from build123d import *

# Parameters (mm, degrees)
SKETCH_1_R          = 2
SKETCH_1_W          = 3
SKETCH_1_H          = 50
EXTRUDE_1_DEPTH     = 10
SKETCH_2_R          = 2
CUT_EXTRUDE_1_DEPTH = 513.83835495


with BuildPart() as part:
    # 스케치1 → 보스-돌출1 (new body)
    with BuildSketch(Plane(origin=(0, 0, 0), x_dir=(1, 0, 0), z_dir=(0, 1, 0))):
        Polygon((-478.203072248, 175), (-448.173072248, 175), (-448.173072248, 185), (-398.173072248, 185), (-398.173072248, 175), (-348.173072248, 175), (-348.173072248, 185), (-298.173072248, 185), (-298.173072248, 175), (-248.173072248, 175), (-248.173072248, 185), (-198.173072248, 185), (-198.173072248, 175), (-148.173072248, 175), (-148.173072248, 185), (-98.173072248, 185), (-98.173072248, 175), (-48.173072248, 175), (-48.173072248, 185), (1.826927752, 185), (1.826927752, 175), (51.826927752, 175), (51.826927752, 185), (101.826927752, 185), (101.826927752, 175), (151.826927752, 175), (151.826927752, 185), (201.826927752, 185), (201.826927752, 175), (207.156927752, 175), (207.156927752, -175), (201.826927752, -175), (201.826927752, -185), (151.826927752, -185), (151.826927752, -175), (101.826927752, -175), (101.826927752, -185), (51.826927752, -185), (51.826927752, -175), (1.826927752, -175), (1.826927752, -185), (-48.173072248, -185), (-48.173072248, -175), (-98.173072248, -175), (-98.173072248, -185), (-148.173072248, -185), (-148.173072248, -175), (-198.173072248, -175), (-198.173072248, -185), (-248.173072248, -185), (-248.173072248, -175), (-298.173072248, -175), (-298.173072248, -185), (-348.173072248, -185), (-348.173072248, -175), (-398.173072248, -175), (-398.173072248, -185), (-448.173072248, -185), (-448.173072248, -175), (-478.203072248, -175), align=None)
        with Locations(Location((-340.173072248, 169, 0), (0, 0, 270))):
            Circle(SKETCH_1_R, mode=Mode.SUBTRACT)
        with Locations(Location((-306.173072248, 169, 0), (0, 0, 270))):
            Circle(SKETCH_1_R, mode=Mode.SUBTRACT)
        with Locations(Location((-290.173072248, 169, 0), (0, 0, 270))):
            Circle(SKETCH_1_R, mode=Mode.SUBTRACT)
        with Locations(Location((-256.173072248, 169, 0), (0, 0, 270))):
            Circle(SKETCH_1_R, mode=Mode.SUBTRACT)
        with Locations(Location((-240.173072248, 169, 0), (0, 0, 270))):
            Circle(SKETCH_1_R, mode=Mode.SUBTRACT)
        with Locations(Location((-206.173072248, 169, 0), (0, 0, 270))):
            Circle(SKETCH_1_R, mode=Mode.SUBTRACT)
        with Locations(Location((-190.173072248, 169, 0), (0, 0, 270))):
            Circle(SKETCH_1_R, mode=Mode.SUBTRACT)
        with Locations(Location((-156.173072248, 169, 0), (0, 0, 270))):
            Circle(SKETCH_1_R, mode=Mode.SUBTRACT)
        with Locations(Location((-140.173072248, 169, 0), (0, 0, 270))):
            Circle(SKETCH_1_R, mode=Mode.SUBTRACT)
        with Locations(Location((-106.173072248, 169, 0), (0, 0, 270))):
            Circle(SKETCH_1_R, mode=Mode.SUBTRACT)
        with Locations(Location((-90.173072248, 169, 0), (0, 0, 270))):
            Circle(SKETCH_1_R, mode=Mode.SUBTRACT)
        with Locations(Location((-56.173072248, 169, 0), (0, 0, 270))):
            Circle(SKETCH_1_R, mode=Mode.SUBTRACT)
        with Locations(Location((-40.173072248, 169, 0), (0, 0, 270))):
            Circle(SKETCH_1_R, mode=Mode.SUBTRACT)
        with Locations(Location((-6.173072248, 169, 0), (0, 0, 270))):
            Circle(SKETCH_1_R, mode=Mode.SUBTRACT)
        with Locations(Location((9.826927752, 169, 0), (0, 0, 270))):
            Circle(SKETCH_1_R, mode=Mode.SUBTRACT)
        with Locations(Location((43.826927752, 169, 0), (0, 0, 270))):
            Circle(SKETCH_1_R, mode=Mode.SUBTRACT)
        with Locations(Location((59.826927752, 169, 0), (0, 0, 270))):
            Circle(SKETCH_1_R, mode=Mode.SUBTRACT)
        with Locations(Location((93.826927752, 169, 0), (0, 0, 270))):
            Circle(SKETCH_1_R, mode=Mode.SUBTRACT)
        with Locations(Location((93.826927752, -169, 0), (0, 0, 90))):
            Circle(SKETCH_1_R, mode=Mode.SUBTRACT)
        with Locations(Location((59.826927752, -169, 0), (0, 0, 90))):
            Circle(SKETCH_1_R, mode=Mode.SUBTRACT)
        with Locations(Location((43.826927752, -169, 0), (0, 0, 90))):
            Circle(SKETCH_1_R, mode=Mode.SUBTRACT)
        with Locations(Location((9.826927752, -169, 0), (0, 0, 90))):
            Circle(SKETCH_1_R, mode=Mode.SUBTRACT)
        with Locations(Location((-6.173072248, -169, 0), (0, 0, 90))):
            Circle(SKETCH_1_R, mode=Mode.SUBTRACT)
        with Locations(Location((-40.173072248, -169, 0), (0, 0, 90))):
            Circle(SKETCH_1_R, mode=Mode.SUBTRACT)
        with Locations(Location((-56.173072248, -169, 0), (0, 0, 90))):
            Circle(SKETCH_1_R, mode=Mode.SUBTRACT)
        with Locations(Location((-90.173072248, -169, 0), (0, 0, 90))):
            Circle(SKETCH_1_R, mode=Mode.SUBTRACT)
        with Locations(Location((-106.173072248, -169, 0), (0, 0, 90))):
            Circle(SKETCH_1_R, mode=Mode.SUBTRACT)
        with Locations(Location((-140.173072248, -169, 0), (0, 0, 90))):
            Circle(SKETCH_1_R, mode=Mode.SUBTRACT)
        with Locations(Location((-156.173072248, -169, 0), (0, 0, 90))):
            Circle(SKETCH_1_R, mode=Mode.SUBTRACT)
        with Locations(Location((-190.173072248, -169, 0), (0, 0, 90))):
            Circle(SKETCH_1_R, mode=Mode.SUBTRACT)
        with Locations(Location((-206.173072248, -169, 0), (0, 0, 90))):
            Circle(SKETCH_1_R, mode=Mode.SUBTRACT)
        with Locations(Location((-240.173072248, -169, 0), (0, 0, 90))):
            Circle(SKETCH_1_R, mode=Mode.SUBTRACT)
        with Locations(Location((-256.173072248, -169, 0), (0, 0, 90))):
            Circle(SKETCH_1_R, mode=Mode.SUBTRACT)
        with Locations(Location((-290.173072248, -169, 0), (0, 0, 90))):
            Circle(SKETCH_1_R, mode=Mode.SUBTRACT)
        with Locations(Location((-306.173072248, -169, 0), (0, 0, 90))):
            Circle(SKETCH_1_R, mode=Mode.SUBTRACT)
        with Locations(Location((-340.173072248, -169, 0), (0, 0, 90))):
            Circle(SKETCH_1_R, mode=Mode.SUBTRACT)
        with Locations(Location((-388.173072248, -163, 0), (0, 0, 270))):
            Circle(SKETCH_1_R, mode=Mode.SUBTRACT)
        with Locations(Location((-358.173072248, -163, 0), (0, 0, 270))):
            Circle(SKETCH_1_R, mode=Mode.SUBTRACT)
        with Locations(Location((-388.173072248, -148, 0), (0, 0, 270))):
            Circle(SKETCH_1_R, mode=Mode.SUBTRACT)
        with Locations(Location((-358.173072248, -148, 0), (0, 0, 270))):
            Circle(SKETCH_1_R, mode=Mode.SUBTRACT)
        with Locations(Location((-388.173072248, -133, 0), (0, 0, 270))):
            Circle(SKETCH_1_R, mode=Mode.SUBTRACT)
        with Locations(Location((-358.173072248, -133, 0), (0, 0, 270))):
            Circle(SKETCH_1_R, mode=Mode.SUBTRACT)
        with Locations(Location((-358.173072248, 163, 0), (0, 0, 90))):
            Circle(SKETCH_1_R, mode=Mode.SUBTRACT)
        with Locations(Location((-388.173072248, 163, 0), (0, 0, 90))):
            Circle(SKETCH_1_R, mode=Mode.SUBTRACT)
        with Locations(Location((-388.173072248, 148, 0), (0, 0, 90))):
            Circle(SKETCH_1_R, mode=Mode.SUBTRACT)
        with Locations(Location((-358.173072248, 148, 0), (0, 0, 90))):
            Circle(SKETCH_1_R, mode=Mode.SUBTRACT)
        with Locations(Location((-358.173072248, 133, 0), (0, 0, 90))):
            Circle(SKETCH_1_R, mode=Mode.SUBTRACT)
        with Locations(Location((-388.173072248, 133, 0), (0, 0, 90))):
            Circle(SKETCH_1_R, mode=Mode.SUBTRACT)
        with Locations(Location((111.826927752, -163, 0), (0, 0, 270))):
            Circle(SKETCH_1_R, mode=Mode.SUBTRACT)
        with Locations(Location((141.826927752, -163, 0), (0, 0, 270))):
            Circle(SKETCH_1_R, mode=Mode.SUBTRACT)
        with Locations(Location((111.826927752, -148, 0), (0, 0, 270))):
            Circle(SKETCH_1_R, mode=Mode.SUBTRACT)
        with Locations(Location((141.826927752, -148, 0), (0, 0, 270))):
            Circle(SKETCH_1_R, mode=Mode.SUBTRACT)
        with Locations(Location((111.826927752, -133, 0), (0, 0, 270))):
            Circle(SKETCH_1_R, mode=Mode.SUBTRACT)
        with Locations(Location((141.826927752, -133, 0), (0, 0, 270))):
            Circle(SKETCH_1_R, mode=Mode.SUBTRACT)
        with Locations(Location((141.826927752, 133, 0), (0, 0, 90))):
            Circle(SKETCH_1_R, mode=Mode.SUBTRACT)
        with Locations(Location((141.826927752, 148, 0), (0, 0, 90))):
            Circle(SKETCH_1_R, mode=Mode.SUBTRACT)
        with Locations(Location((141.826927752, 163, 0), (0, 0, 90))):
            Circle(SKETCH_1_R, mode=Mode.SUBTRACT)
        with Locations(Location((111.826927752, 163, 0), (0, 0, 90))):
            Circle(SKETCH_1_R, mode=Mode.SUBTRACT)
        with Locations(Location((111.826927752, 148, 0), (0, 0, 90))):
            Circle(SKETCH_1_R, mode=Mode.SUBTRACT)
        with Locations(Location((111.826927752, 133, 0), (0, 0, 90))):
            Circle(SKETCH_1_R, mode=Mode.SUBTRACT)
        with Locations((-166.673072248, 100)):
            Rectangle(SKETCH_1_W, SKETCH_1_H, mode=Mode.SUBTRACT)
        with Locations((-166.673072248, 0)):
            Rectangle(SKETCH_1_W, SKETCH_1_H, mode=Mode.SUBTRACT)
        with Locations((-166.673072248, -100)):
            Rectangle(SKETCH_1_W, SKETCH_1_H, mode=Mode.SUBTRACT)
        with Locations((-399.473072248, 100)):
            Rectangle(SKETCH_1_W, SKETCH_1_H, mode=Mode.SUBTRACT)
        with Locations((-399.473072248, 0)):
            Rectangle(SKETCH_1_W, SKETCH_1_H, mode=Mode.SUBTRACT)
        with Locations((-399.473072248, -100)):
            Rectangle(SKETCH_1_W, SKETCH_1_H, mode=Mode.SUBTRACT)
    extrude(amount=EXTRUDE_1_DEPTH)

    # 스케치2 → 컷-돌출1 (cut, through all)
    with BuildSketch(Plane(origin=(0, 10, 0), x_dir=(1, 0, 0), z_dir=(0, 1, 0))):
        with Locations(Location((137.156927752, 30, 0), (0, 0, 270))):
            Circle(SKETCH_2_R)
        with Locations(Location((187.156927752, 30, 0), (0, 0, 270))):
            Circle(SKETCH_2_R)
        with Locations(Location((-65.173072248, 30, 0), (0, 0, 270))):
            Circle(SKETCH_2_R)
        with Locations(Location((-65.173072248, -30, 0), (0, 0, 90))):
            Circle(SKETCH_2_R)
        with Locations(Location((187.156927752, -30, 0), (0, 0, 90))):
            Circle(SKETCH_2_R)
        with Locations(Location((137.156927752, -30, 0), (0, 0, 90))):
            Circle(SKETCH_2_R)
    extrude(amount=-CUT_EXTRUDE_1_DEPTH, mode=Mode.SUBTRACT)


solid = part.part
Can you work these out from the model? Positions are in its coordinate system, mm. Give positions to 0.01 mm unless a question says otherwise; leave off trailing zeros. Write each loop counter-clockwise with the first axis right and the second up, starting at its lowest first coordinate (ties: lowest second). Pieces come first, ordered by that corner, then holes. Notation, with made-up numbers: (43.25, 0.25) -> (85.25, 0.25) arc R19 cw to (85.25, 21.25) -> close; hole circle Ø1 at (16.25, 39). An arc over 180 degrees is marked (long way). Answer as a JSON object with one key per item and string values. Group by question number.
Item 1: I'm going to push flat-ended pins straight in: P1, Ø1.5, axis at x = 126.5, y = 7, coming from the +Z side; P2, Ø5, axis at y = 5.5, z = -178.5, coming from the +X side. Where does each tip first touch, or does it pass through?
Item 2: Please list where these lines run through material, in increasing order: line 1 (X direction, y = 6.25, z = 99); line 2 (X direction, y = 5.5, z = -133); line 3 (Z direction, x = 150.5, y = 5.5). Write a range as [from, to].
Item 3: Suppose I cut it at A-A (x = -377). Please give me the cut outline in (y, z).
Item 4: Suppose I cut it at B-B (y = 6.75). State how many separate pieces and enclosed holes the cut face has, plus the area to 3 significant figures.
Findings:
{
 "1": {"P1": "stops at z = 175", "P2": "stops at x = 201.83"},
 "2": {"line 1": "x = [-478.2, -400.97], [-397.97, -168.17], [-165.17, 207.16]", "line 2": "x = [-478.2, -390.17], [-386.17, -360.17], [-356.17, 109.83], [113.83, 139.83], [143.83, 207.16]", "line 3": "z = [-175, 175]"},
 "3": {"outline": "(0, -175) -> (10, -175) -> (10, 175) -> (0, 175) -> close"},
 "4": {"separate pieces": "1", "enclosed holes": "72", "area": "245,000 mm²"}
}
